Geometry check sheet. Reference: the model listing, model coordinates, mm. A direction names the side the tool comes from. Round coordinates to 2 decimals unless told otherwise and drop trailing zeros. Write each loop counter-clockwise with the first axis right and the second up, starting at its lowest first coordinate (ties: lowest second). Pieces come first, ordered by that corner, then holes. Notation, with made-up numbers: M 67,0.5 L 86,0.5 A15 cw 86,13.5 Z; hole C 71,52.25 d6. An arc over 180 degrees is marked long. Answer as CSV lines item,"result". Start each with the question number.
```python
from build123d import *

# Parameters (mm, degrees)
F0_R     = 11.2522
F1_DEPTH = 7.62
F2_DEPTH = 5.334


with BuildPart() as f1:
    # F0 (on Top) → F1 (new body)
    with BuildSketch(Plane.XY):
        with BuildLine():
            ThreePointArc((12.7369944105, -2.4049880816), (12.9056707985, -1.2077481218), (12.962059801, 0))
            ThreePointArc((12.962059801, 0), (9.9385595014, 8.321059387), (2.2785680744, 12.7602163702))
            ThreePointArc((2.2785680744, 12.7602163702), (0, 12.5583729394), (-2.2785680744, 12.7602163702))
            ThreePointArc((-2.2785680744, 12.7602163702), (-10.6706436404, 7.3588286149), (-12.7369944105, -2.4049880816))
            ThreePointArc((-12.7369944105, -2.4049880816), (-10.231616704, -5.6270418202), (-8.8523481214, -9.4684173452))
            ThreePointArc((-8.8523481214, -9.4684173452), (0, -12.962059801), (8.8523481214, -9.4684173452))
            ThreePointArc((8.8523481214, -9.4684173452), (10.231616704, -5.6270418202), (12.7369944105, -2.4049880816))
        make_face()
        Circle(F0_R, mode=Mode.SUBTRACT)
        with BuildLine():
            ThreePointArc((-2.2785680744, 12.7602163702), (0, 12.5583729394), (2.2785680744, 12.7602163702))
            ThreePointArc((2.2785680744, 12.7602163702), (0, 12.962059801), (-2.2785680744, 12.7602163702))
        make_face()
        with BuildLine():
            ThreePointArc((-2.2785680744, 12.7602163702), (0, 12.962059801), (2.2785680744, 12.7602163702))
            ThreePointArc((2.2785680744, 12.7602163702), (9.9385595014, 17.1993733535), (12.962059801, 25.5204327404))
            ThreePointArc((12.962059801, 25.5204327404), (12.6382642104, 28.3995423305), (11.6830544332, 31.1348101232))
            ThreePointArc((11.6830544332, 31.1348101232), (6.9007644107, 36.492872981), (0, 38.4824925414))
            ThreePointArc((0, 38.4824925414), (-12.9115003379, 26.6641780399), (-2.2785680744, 12.7602163702))
        make_face()
        with Locations((0, 25.5204327404)):
            Circle(F0_R, mode=Mode.SUBTRACT)
        with BuildLine():
            ThreePointArc((34.5514023329, -11.8734054267), (26.7502692198, 0.0169196322), (12.7369944105, -2.4049880816))
            ThreePointArc((12.7369944105, -2.4049880816), (11.3577258278, -6.2463636065), (8.8523481214, -9.4684173452))
            ThreePointArc((8.8523481214, -9.4684173452), (11.4621329747, -19.9638084371), (21.1220092921, -24.8270378875))
            ThreePointArc((21.1220092921, -24.8270378875), (27.8669248008, -23.2139060833), (32.8148156049, -18.3544353272))
            ThreePointArc((32.8148156049, -18.3544353272), (33.0812954491, -17.869238349), (33.3268161418, -17.373106104))
            ThreePointArc((33.3268161418, -17.373106104), (34.2415524007, -14.6905990161), (34.5514023329, -11.8734054267))
        make_face()
        with Locations((21.5893425319, -11.8734054267)):
            Circle(F0_R, mode=Mode.SUBTRACT)
        with BuildLine():
            ThreePointArc((8.8523481214, -9.4684173452), (11.3577258278, -6.2463636065), (12.7369944105, -2.4049880816))
            ThreePointArc((12.7369944105, -2.4049880816), (10.231616704, -5.6270418202), (8.8523481214, -9.4684173452))
        make_face()
        with BuildLine():
            ThreePointArc((-8.8523481214, -9.4684173452), (-10.231616704, -5.6270418202), (-12.7369944105, -2.4049880816))
            ThreePointArc((-12.7369944105, -2.4049880816), (-11.3577258278, -6.2463636065), (-8.8523481214, -9.4684173452))
        make_face()
        with BuildLine():
            ThreePointArc((-8.8523481214, -9.4684173452), (-11.3577258278, -6.2463636065), (-12.7369944105, -2.4049880816))
            ThreePointArc((-12.7369944105, -2.4049880816), (-23.1489478225, 0.9944858388), (-32.4473199354, -4.7939053745))
            ThreePointArc((-32.4473199354, -4.7939053745), (-34.5466450824, -11.5222574559), (-32.8148156049, -18.3544353272))
            ThreePointArc((-32.8148156049, -18.3544353272), (-18.2345145916, -24.3937937504), (-8.6272827309, -11.8734054267))
            ThreePointArc((-8.6272827309, -11.8734054267), (-8.6836717334, -10.665657305), (-8.8523481214, -9.4684173452))
        make_face()
        with Locations((-21.5893425319, -11.8734054267)):
            Circle(F0_R, mode=Mode.SUBTRACT)
        with BuildLine():
            ThreePointArc((33.5095214822, 28.6722648172), (18.313797705, 38.902696715), (0, 38.4824925414))
            ThreePointArc((0, 38.4824925414), (6.9007644107, 36.492872981), (11.6830544332, 31.1348101232))
            ThreePointArc((11.6830544332, 31.1348101232), (23.0045235804, 33.5218836362), (33.5095214822, 28.6722648172))
        make_face()
        with BuildLine():
            ThreePointArc((32.8148156049, -18.3544353272), (27.8669248008, -23.2139060833), (21.1220092921, -24.8270378875))
            ThreePointArc((21.1220092921, -24.8270378875), (17.5285410214, -35.8252545336), (8.0761489747, -42.4980401738))
            ThreePointArc((8.0761489747, -42.4980401738), (24.3755164942, -34.6034732765), (33.2400792742, -18.8106554549))
            ThreePointArc((33.2400792742, -18.8106554549), (33.0293167827, -18.5808028908), (32.8148156049, -18.3544353272))
        make_face()
        with BuildLine():
            Line((33.2400792742, -18.8106554549), (33.3268161418, -17.373106104))
            ThreePointArc((33.3268161418, -17.373106104), (33.0812954491, -17.869238349), (32.8148156049, -18.3544353272))
            ThreePointArc((32.8148156049, -18.3544353272), (33.0293167827, -18.5808028908), (33.2400792742, -18.8106554549))
        make_face()
        with BuildLine():
            ThreePointArc((-32.8148156049, -18.3544353272), (-34.5466450824, -11.5222574559), (-32.4473199354, -4.7939053745))
            ThreePointArc((-32.4473199354, -4.7939053745), (-39.8779765619, 3.7961234456), (-40.8424568889, 15.1130590171))
            ThreePointArc((-40.8424568889, 15.1130590171), (-42.2015912045, -2.7503305518), (-33.2137545387, -18.2476440302))
            ThreePointArc((-33.2137545387, -18.2476440302), (-33.0145748071, -18.3021220393), (-32.8148156049, -18.3544353272))
        make_face()
    extrude(amount=F1_DEPTH)

    # F0 (on Top) → F2 (join)
    with BuildSketch(Plane.XY):
        with BuildLine():
            ThreePointArc((32.8148156049, -18.3544353272), (27.8669248008, -23.2139060833), (21.1220092921, -24.8270378875))
            ThreePointArc((21.1220092921, -24.8270378875), (17.5285410214, -35.8252545336), (8.0761489747, -42.4980401738))
            ThreePointArc((8.0761489747, -42.4980401738), (24.3755164942, -34.6034732765), (33.2400792742, -18.8106554549))
            ThreePointArc((33.2400792742, -18.8106554549), (33.0293167827, -18.5808028908), (32.8148156049, -18.3544353272))
        make_face()
        with BuildLine():
            ThreePointArc((-32.8148156049, -18.3544353272), (-34.5466450824, -11.5222574559), (-32.4473199354, -4.7939053745))
            ThreePointArc((-32.4473199354, -4.7939053745), (-39.8779765619, 3.7961234456), (-40.8424568889, 15.1130590171))
            ThreePointArc((-40.8424568889, 15.1130590171), (-42.2015912045, -2.7503305518), (-33.2137545387, -18.2476440302))
            ThreePointArc((-33.2137545387, -18.2476440302), (-33.0145748071, -18.3021220393), (-32.8148156049, -18.3544353272))
        make_face()
        with BuildLine():
            ThreePointArc((33.5095214822, 28.6722648172), (18.313797705, 38.902696715), (0, 38.4824925414))
            ThreePointArc((0, 38.4824925414), (6.9007644107, 36.492872981), (11.6830544332, 31.1348101232))
            ThreePointArc((11.6830544332, 31.1348101232), (23.0045235804, 33.5218836362), (33.5095214822, 28.6722648172))
        make_face()
        with BuildLine():
            ThreePointArc((-2.2785680744, 12.7602163702), (0, 12.962059801), (2.2785680744, 12.7602163702))
            ThreePointArc((2.2785680744, 12.7602163702), (9.9385595014, 17.1993733535), (12.962059801, 25.5204327404))
            ThreePointArc((12.962059801, 25.5204327404), (12.6382642104, 28.3995423305), (11.6830544332, 31.1348101232))
            ThreePointArc((11.6830544332, 31.1348101232), (6.9007644107, 36.492872981), (0, 38.4824925414))
            ThreePointArc((0, 38.4824925414), (-12.9115003379, 26.6641780399), (-2.2785680744, 12.7602163702))
        make_face()
        with Locations((0, 25.5204327404)):
            Circle(F0_R, mode=Mode.SUBTRACT)
        with BuildLine():
            ThreePointArc((12.7369944105, -2.4049880816), (12.9056707985, -1.2077481218), (12.962059801, 0))
            ThreePointArc((12.962059801, 0), (9.9385595014, 8.321059387), (2.2785680744, 12.7602163702))
            ThreePointArc((2.2785680744, 12.7602163702), (0, 12.5583729394), (-2.2785680744, 12.7602163702))
            ThreePointArc((-2.2785680744, 12.7602163702), (-10.6706436404, 7.3588286149), (-12.7369944105, -2.4049880816))
            ThreePointArc((-12.7369944105, -2.4049880816), (-10.231616704, -5.6270418202), (-8.8523481214, -9.4684173452))
            ThreePointArc((-8.8523481214, -9.4684173452), (0, -12.962059801), (8.8523481214, -9.4684173452))
            ThreePointArc((8.8523481214, -9.4684173452), (10.231616704, -5.6270418202), (12.7369944105, -2.4049880816))
        make_face()
        Circle(F0_R, mode=Mode.SUBTRACT)
        with BuildLine():
            ThreePointArc((34.5514023329, -11.8734054267), (26.7502692198, 0.0169196322), (12.7369944105, -2.4049880816))
            ThreePointArc((12.7369944105, -2.4049880816), (11.3577258278, -6.2463636065), (8.8523481214, -9.4684173452))
            ThreePointArc((8.8523481214, -9.4684173452), (11.4621329747, -19.9638084371), (21.1220092921, -24.8270378875))
            ThreePointArc((21.1220092921, -24.8270378875), (27.8669248008, -23.2139060833), (32.8148156049, -18.3544353272))
            ThreePointArc((32.8148156049, -18.3544353272), (33.0812954491, -17.869238349), (33.3268161418, -17.373106104))
            ThreePointArc((33.3268161418, -17.373106104), (34.2415524007, -14.6905990161), (34.5514023329, -11.8734054267))
        make_face()
        with Locations((21.5893425319, -11.8734054267)):
            Circle(F0_R, mode=Mode.SUBTRACT)
        with BuildLine():
            ThreePointArc((8.8523481214, -9.4684173452), (11.3577258278, -6.2463636065), (12.7369944105, -2.4049880816))
            ThreePointArc((12.7369944105, -2.4049880816), (10.231616704, -5.6270418202), (8.8523481214, -9.4684173452))
        make_face()
        with BuildLine():
            ThreePointArc((-2.2785680744, 12.7602163702), (0, 12.5583729394), (2.2785680744, 12.7602163702))
            ThreePointArc((2.2785680744, 12.7602163702), (0, 12.962059801), (-2.2785680744, 12.7602163702))
        make_face()
        with BuildLine():
            ThreePointArc((-8.8523481214, -9.4684173452), (-10.231616704, -5.6270418202), (-12.7369944105, -2.4049880816))
            ThreePointArc((-12.7369944105, -2.4049880816), (-11.3577258278, -6.2463636065), (-8.8523481214, -9.4684173452))
        make_face()
        with BuildLine():
            ThreePointArc((-8.8523481214, -9.4684173452), (-11.3577258278, -6.2463636065), (-12.7369944105, -2.4049880816))
            ThreePointArc((-12.7369944105, -2.4049880816), (-23.1489478225, 0.9944858388), (-32.4473199354, -4.7939053745))
            ThreePointArc((-32.4473199354, -4.7939053745), (-34.5466450824, -11.5222574559), (-32.8148156049, -18.3544353272))
            ThreePointArc((-32.8148156049, -18.3544353272), (-18.2345145916, -24.3937937504), (-8.6272827309, -11.8734054267))
            ThreePointArc((-8.6272827309, -11.8734054267), (-8.6836717334, -10.665657305), (-8.8523481214, -9.4684173452))
        make_face()
        with Locations((-21.5893425319, -11.8734054267)):
            Circle(F0_R, mode=Mode.SUBTRACT)
    extrude(amount=F2_DEPTH)


solid = f1.part
```
1) Mould release check, pull along X, two halves, no side actions. Record for faces 1 (the cylindrical face through (18.56, 38.83, 3.76)), 2 (the cylindrical face through (-42.257, -2.502, 3.757)), 3 (the cylindrical face through (22.84, 33.54, 3.76)), 4 (the cylindrical face through (-1.465, 11.156, 3.757)): released by +X, released by -X, zero draft, split by the parting line, or undercut.
2) Section check C-C, the plane z = 4.75. Record the cut outline in (x, y).
3) Go/stop test with flat-tipped pins: pin 1 (13.5 mm diameter, centred on x = 0, y = 0, fed in from -Z); pin 2 (1 mm diameter, centred on x = 2.5, z = 5.5, fed in from -Y); pin 3 (3 mm diameter, centred on x = -16, z = 2, fed in from +Y). Record where each tip stops, or that it passes through.
4) Section check A-A, the plane x = 26. Record the cut outline in (y, z), plus the area to 3 significant figures.
5) Access from +Z, -Z, +X, -X, +Y, -Y to the whole of each face (thin tool, end or side, straight path). Record for faces 5 (the cylindrical face through (-39.815, 3.647, 3.757)), 6 (the flat face through (4, 11, 0)).
6) Scan lines: line 1 (Y direction, x = 1, z = 0.5); line 2 (Y direction, x = -22, z = 3.75); line 3 (Y direction, x = 17, z = 4.5). Record each from-to range of solid material in increasing order. Write a range as from..to.
7) Section check D-D, the plane x = 16.5. Record the cut outline in (y, z), plus the area to 3 significant figures.
8) Section check B-B, the plane y = 10. Record the cut outline in (x, z).
Results:
1,face 1,"split by the parting line"
1,face 2,"released by -X"
1,face 3,"undercut"
1,face 4,"undercut"
2,outline,"M -40.84,15.11 A30.24 ccw -33.21,-18.25 A19.03 ccw -32.81,-18.35 A12.96 ccw -8.85,-9.47 A12.96 ccw 8.85,-9.47 A12.96 ccw 21.12,-24.83 A18.38 cw 8.08,-42.5 A30.24 ccw 33.24,-18.81 L 33.33,-17.37 A12.96 ccw 12.74,-2.4 A12.96 ccw 2.28,12.76 A12.96 ccw 11.68,31.13 A18.38 cw 33.51,28.67 A30.24 ccw 0,38.48 A12.96 ccw -2.28,12.76 A12.96 ccw -12.74,-2.4 A12.96 ccw -32.45,-4.79 A18.38 cw Z; hole C -21.59,-11.87 d22.5; hole C 0,0 d22.5; hole C 0,25.52 d22.5; hole C 21.59,-11.87 d22.5"
3,pin 1,"passes through"
3,pin 2,"stops at y = -12.81"
3,pin 3,"stops at y = 0.43"
4,outline,"M -32.95,0 L -22.23,0 L -22.23,7.62 L -32.95,7.62 Z; M -1.52,0 L 0.32,0 L 0.32,7.62 L -1.52,7.62 Z; M 32.93,0 L 35.43,0 L 35.43,7.62 L 32.93,7.62 Z"
4,area,"115 mm^2"
5,face 5,"+Z, -Z"
5,face 6,"-Z, +X, -X, +Y, -Y"
6,line 1,"y = -12.92..-11.21, 11.21..14.31, 36.73..38.81"
6,line 2,"y = -24.83..-23.12, -0.63..1.08"
6,line 3,"y = -39.72..-36.51, -24..-22.15, -1.6..0.25, 33.21..39.26"
7,outline,"M -39.96,0 L -37.1,0 L -37.1,7.62 L -39.96,7.62 Z; M -23.79,0 L -21.91,0 L -21.91,7.62 L -23.79,7.62 Z; M -1.84,0 L 0.05,0 L 0.05,7.62 L -1.84,7.62 Z; M 33.09,0 L 39.37,0 L 39.37,7.62 L 33.09,7.62 Z"
7,area,"98.4 mm^2"
8,outline,"M -42.36,0 L -41.3,0 L -41.3,7.62 L -42.36,7.62 Z; M -8.25,0 L -5.16,0 L -5.16,7.62 L -8.25,7.62 Z; M 5.16,0 L 8.25,0 L 8.25,7.62 L 5.16,7.62 Z"
